```python
from build123d import *

# Parameters (mm, degrees)
ESQUISSE1_W        = 20
ESQUISSE1_H        = 20
ESQUISSE1_R        = 1
ESQUISSE1_R_2      = 3.25
BOSS_EXTRU_1_DEPTH = 40


with BuildPart() as part:
    # Esquisse1 → Boss.-Extru.1 (new body)
    with BuildSketch(Plane(origin=(0, 0, 0), x_dir=(1, 0, 0), z_dir=(0, 1, 0))):
        Rectangle(ESQUISSE1_W, ESQUISSE1_H)
        with Locations(Location((-5.303300859, 5.303300859, 0), (0, 0, 270))):
            Circle(ESQUISSE1_R, mode=Mode.SUBTRACT)
        with Locations(Location((5.303300859, -5.303300859, 0), (0, 0, 90))):
            Circle(ESQUISSE1_R, mode=Mode.SUBTRACT)
        with Locations(Location((0, 0, 0), (0, 0, 270))):
            Circle(ESQUISSE1_R_2, mode=Mode.SUBTRACT)
    extrude(amount=-BOSS_EXTRU_1_DEPTH)


solid = part.part
```
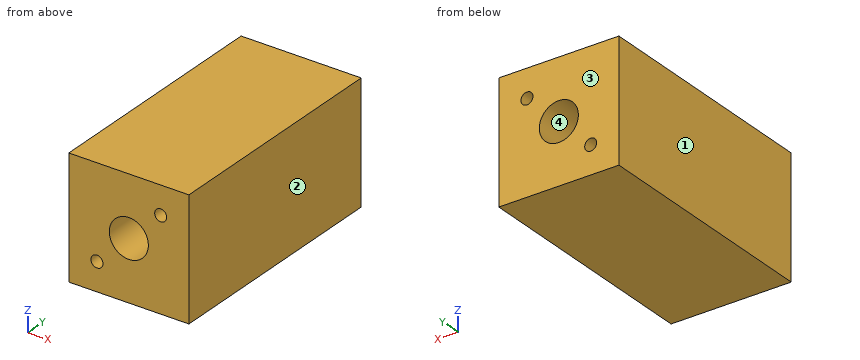
Geometry check sheet. Reference: the model listing, model coordinates, mm. Face numbers are marked on the shaded views. Round coordinates to 2 decimals unless told otherwise and drop trailing zeros. Order: outer loops, then holes, each group sorted by start corner. A loop starts at its lowest first (then second) coordinate and runs counter-clockwise, first axis right, second up. Notation, with made-up numbers: (40.25, 58.5) -> (75.25, 58.5) arc R24 cw to (75.25, 80.5) -> close; hole circle Ø10 at (14.5, 57). An arc over 180 degrees is marked (long way). Return JSON: item names as keys, results as strings. Group by question number.
Q1. Release check for a two-part mould opening along X. For the marked faces 1, 2, 3 and 4 record: released by +X, released by -X, zero draft, split by the parting line, or undercut.
Q2. Section check B-B, the plane z = 0. Record the boundary of the cut face in (x, y), plus the area to 3 significant figures.
Q3. Material ranges on probe 1 along X at (y, z) = (-29.5, 0); probe 2 along X at (y, z) = (-22, -5.75); probe 3 along Z at (x, y) = (-0.75, -14.5), recorded low to high. Write a range as from..to.
Q4. Gauge pin test, flat end, axial feed: pin 1 (6 mm diameter, centred on x = 0, z = 0, fed in from +Y) (1 decimal). Record the tip position at first contact, or that the pin passes through.
Q5. Section check A-A, the plane x = 0. Record the boundary of the cut face in (y, z).
Q6. Section check C-C, the plane y = -16. Record the boundary of the cut face in (x, z), plus the area to 3 significant figures.
Numbers:
{
 "1": {"face 1": "released by -X", "face 2": "released by +X", "face 3": "zero draft", "face 4": "undercut"},
 "2": {"outline": "(-10, -40) -> (-3.25, -40) -> (-3.25, 0) -> (-10, 0) -> close; (3.25, -40) -> (10, -40) -> (10, 0) -> (3.25, 0) -> close", "area": "540 mm^2"},
 "3": {"probe 1": "-10..-3.25, 3.25..10", "probe 2": "-10..-6.2, -4.41..10", "probe 3": "-10..-3.16, 3.16..10"},
 "4": {"pin 1": "through"},
 "5": {"outline": "(-40, -10) -> (0, -10) -> (0, -3.25) -> (-40, -3.25) -> close; (-40, 3.25) -> (0, 3.25) -> (0, 10) -> (-40, 10) -> close"},
 "6": {"outline": "(-10, -10) -> (10, -10) -> (10, 10) -> (-10, 10) -> close; hole circle Ø2 at (-5.3, -5.3); hole circle Ø6.5 at (0, 0); hole circle Ø2 at (5.3, 5.3)", "area": "361 mm^2"}
}
